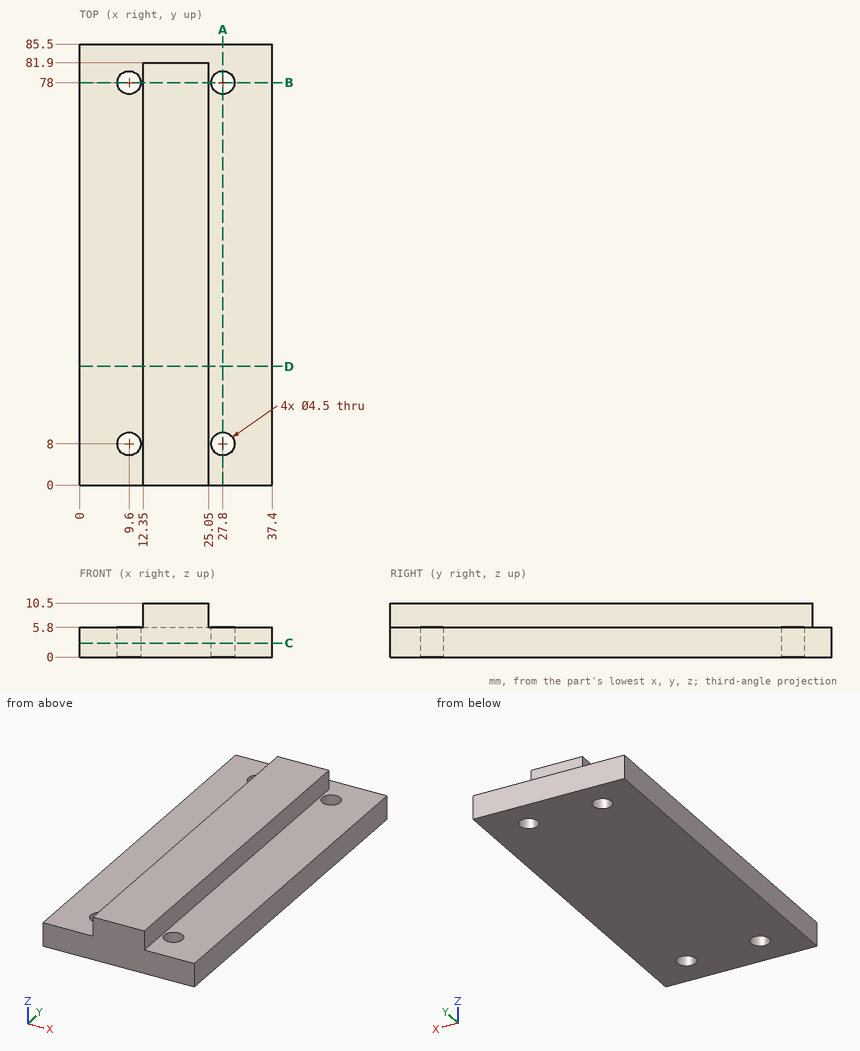
Could you check a few things on this drawing? It's one solid part, dimensions in mm from its lowest x, y, z. Coordinates: 2 decimals unless noted, no trailing zeros. Order: outer loops, then holes, each group sorted by start corner. A loop starts at its lowest first (then second) coordinate and runs counter-clockwise, first axis right, second up.
1) I need wall thicknesses on line 1 (Y direction, x = 9.6, z = 4); line 2 (Y direction, x = 11, z = 5.25); line 3 (Z direction, x = 9, y = 21.5). Which ranges of each line are inside material? Lowest first, please.
2) Imagine slicing it at A-A on x = 27.8. List the corners of the cut face in (y, z) for me.
3) Imagine slicing it at B-B on y = 78. List the corners of the cut face in (x, z) for me.
4) Will these pins go through, and if not, where does the flat tip stop? pin 1 (5 mm diameter, centred on x = 27.8, y = 8, fed in from +Z); pin 2 (4 mm diameter, centred on x = 17, z = 8, fed in from +Y); pin 3 (4 mm diameter, centred on x = 9.6, y = 78, fed in from -Z); pin 4 (2.5 mm diameter, centred on y = 24.5, z = 8, fed in from -X).
5) Imagine slicing it at C-C on z = 2.75. List the corners of the cut face in (x, y) for me, and give its area (3 significant figures).
6) Imagine slicing it at D-D on y = 23. List the corners of the cut face in (x, z) for me, and give its area (3 significant figures).
Response values:
1. line 1: y = 0 to 5.75, 10.25 to 75.75, 80.25 to 85.5
1. line 2: y = 0 to 6.24, 9.76 to 76.24, 79.76 to 85.5
1. line 3: z = 0 to 5.8
2. outline: (0, 0) - (5.75, 0) - (5.75, 5.8) - (0, 5.8) - close; (10.25, 0) - (75.75, 0) - (75.75, 5.8) - (10.25, 5.8) - close; (80.25, 0) - (85.5, 0) - (85.5, 5.8) - (80.25, 5.8) - close
3. outline: (0, 0) - (7.35, 0) - (7.35, 5.8) - (0, 5.8) - close; (11.85, 0) - (25.55, 0) - (25.55, 5.8) - (25.05, 5.8) - (25.05, 10.5) - (12.35, 10.5) - (12.35, 5.8) - (11.85, 5.8) - close; (30.05, 0) - (37.4, 0) - (37.4, 5.8) - (30.05, 5.8) - close
4. pin 1: stops at z = 5.8
4. pin 2: stops at y = 81.9
4. pin 3: passes through
4. pin 4: stops at x = 12.35
5. outline: (0, 0) - (37.4, 0) - (37.4, 85.5) - (0, 85.5) - close; hole circle Ø4.5 at (9.6, 8); hole circle Ø4.5 at (9.6, 78); hole circle Ø4.5 at (27.8, 8); hole circle Ø4.5 at (27.8, 78)
5. area: 3,130 mm2
6. outline: (0, 0) - (37.4, 0) - (37.4, 5.8) - (25.05, 5.8) - (25.05, 10.5) - (12.35, 10.5) - (12.35, 5.8) - (0, 5.8) - close
6. area: 277 mm2
